The listing builds one solid part. Answer for the finished solid, in the listing's coordinates (mm). A direction names the side the tool comes from. Give positions to 0.01 mm unless a question says otherwise; leave off trailing zeros. Write each loop counter-clockwise with the first axis right and the second up, starting at its lowest first coordinate (ties: lowest second). Pieces come first, ordered by that corner, then holes. Notation, with made-up numbers: (16.5, 54.25) - (71.5, 54.25) arc R20 ccw to (71.5, 88.25) - close; hole circle Ø4 at (78.25, 51). An arc over 180 degrees is marked (long way). Answer as CSV lines item,"result". Start each with the question number.
(1) For a pull along X with two mould halves and no side action, classify faces 3 (the face through (-58.426, -20.504, 2.095)), 4 (the face through (98.802, -3.549, 2.095)), 5 (the face through (-79, 0, 2)), 6 (the face through (-102.5, -20, 2)) as pulls with the +X half, pulls with the -X half, needs draft (parallel to the pull), parting line crosses it, or undercut.
(2) Find section B-B (z = 1.7). State how many separate pieces and enclosed holes the cut face has, then the cut area to 3 significant figures.
(3) Find section C-C (x = 35). Write down the section's boundary in (y, z).
(4) Find section A-A (x = -73.4). Write down the section's boundary in (y, z).
(5) Straight lines are drawn through the part: probe 1 along Y at (x, z) = (79.5, 2.5); probe 2 along X at (y, z) = (-39.5, 0.4); probe 3 along X at (y, z) = (-10, 1). For each, find the intervals that lie inside material, in ascending order.
(6) For faces 1 (the face through (97.43, -41.62, 2.1)), 2 (the face through (58.084, -5.67, 2.095)), determine the directions among +Z, -Z, +X, -X, +Y, -Y from which every point of the face is accessible in a straight line to the end or side of a thin tool.
(7) This flat-tipped pin is pushed along its axis until it touches: pin 1 Ø1.5 at (x, z) = (-58, 1.5) entering from +Y. Where does it stop, or does it pass through?
from build123d import *

# Parameters (mm, degrees)
SKETCH1_R           = 2.500008074
SKETCH1_R_2         = 2.499971378
SKETCH1_R_3         = 1.650003804
SKETCH1_R_4         = 1.64998699
SKETCH1_R_5         = 2.498738291
SKETCH1_R_6         = 2.499947604
SKETCH1_R_7         = 1.499976694
SKETCH1_R_8         = 1.500017827
SKETCH1_R_9         = 1.50001874
SKETCH1_R_10        = 1.499989662
BOSS_EXTRUDE1_DEPTH = 4.25


with BuildPart() as part:
    # Sketch1 → Boss-Extrude1 (new body)
    with BuildSketch(Plane.XY):
        Polygon((102.5, -33), (102.5, -7), (95, 0), (64, 0), (52, -11.5), (-52, -11.5), (-64, 0), (-95, 0), (-102.5, -7), (-102.5, -33), (-92.5, -50), (92.5, -50), align=None)
        with Locations((-96.600008074, -9.899995929)):
            Circle(SKETCH1_R, mode=Mode.SUBTRACT)
        with Locations((-73.4, -9.899975)):
            Circle(SKETCH1_R_2, mode=Mode.SUBTRACT)
        with Locations((-59.99995, -20.999975175)):
            Circle(SKETCH1_R_3, mode=Mode.SUBTRACT)
        with Locations((-59.99995, -32.000038683)):
            Circle(SKETCH1_R_4, mode=Mode.SUBTRACT)
        with Locations((-73.398707193, -33.112466424)):
            Circle(SKETCH1_R_5, mode=Mode.SUBTRACT)
        with Locations((-96.597049433, -33.113350272)):
            Circle(SKETCH1_R_6, mode=Mode.SUBTRACT)
        with Locations((-90.500019389, -40)):
            Circle(SKETCH1_R_7, mode=Mode.SUBTRACT)
        with Locations((-79.5, -40)):
            Circle(SKETCH1_R_8, mode=Mode.SUBTRACT)
        with Locations((0.003309528, -20.00748325)):
            Circle(SKETCH1_R_9, mode=Mode.SUBTRACT)
        with Locations((0.003345163, -46.007511034)):
            Circle(SKETCH1_R_10, mode=Mode.SUBTRACT)
        with Locations(Location((96.606599424, -9.899731124, 0), (0, 0, 180))):
            Circle(SKETCH1_R, mode=Mode.SUBTRACT)
        with Locations(Location((96.603704415, -33.113085476, 0), (0, 0, 180))):
            Circle(SKETCH1_R_6, mode=Mode.SUBTRACT)
        with Locations(Location((90.506693248, -39.999751917, 0), (0, 0, 180))):
            Circle(SKETCH1_R_7, mode=Mode.SUBTRACT)
        with Locations(Location((73.40659135, -9.899773791, 0), (0, 0, 180))):
            Circle(SKETCH1_R_2, mode=Mode.SUBTRACT)
        with Locations(Location((79.506673859, -39.999782069, 0), (0, 0, 180))):
            Circle(SKETCH1_R_8, mode=Mode.SUBTRACT)
        with Locations(Location((73.405362172, -33.112265218, 0), (0, 0, 180))):
            Circle(SKETCH1_R_5, mode=Mode.SUBTRACT)
        with Locations(Location((60.006571777, -20.999810697, 0), (0, 0, 180))):
            Circle(SKETCH1_R_3, mode=Mode.SUBTRACT)
        with Locations(Location((60.00660193, -31.999874205, 0), (0, 0, 180))):
            Circle(SKETCH1_R_4, mode=Mode.SUBTRACT)
    extrude(amount=BOSS_EXTRUDE1_DEPTH)


solid = part.part
Result set:
1,face 3,"undercut"
1,face 4,"pulls with the +X half"
1,face 5,"needs draft"
1,face 6,"pulls with the -X half"
2,separate pieces,"1"
2,enclosed holes,"18"
2,area,"8,460 mm^2"
3,outline,"(-50, 0) - (-11.5, 0) - (-11.5, 4.25) - (-50, 4.25) - close"
4,outline,"(-50, 0) - (-35.61, 0) - (-35.61, 4.25) - (-50, 4.25) - close; (-30.61, 0) - (-12.4, 0) - (-12.4, 4.25) - (-30.61, 4.25) - close; (-7.4, 0) - (0, 0) - (0, 4.25) - (-7.4, 4.25) - close"
5,probe 1,"-50 to -41.5, -38.5 to 0"
5,probe 2,"-98.68 to -91.91, -89.09 to -80.91, -78.09 to 78.09, 80.92 to 89.09, 91.92 to 98.68"
5,probe 3,"-102.5 to -99.1, -94.1 to -75.9, -70.9 to -53.57, 53.57 to 70.91, 75.9 to 94.11, 99.1 to 102.5"
6,face 1,"+Z, -Z, +X, -Y"
6,face 2,"+Z, -Z, +Y"
7,pin 1,"y = -5.03"
